```python
from build123d import *

# Parameters (mm, degrees)
SKETCH1_W           = 63.5
SKETCH1_H           = 63.5
BOSS_EXTRUDE1_DEPTH = 1.5875
FILLET1_R           = 0.508
FILLET2_R           = 3.175


with BuildPart() as part:
    # Sketch1 → Boss-Extrude1 (new body)
    with BuildSketch(Plane(origin=(0, 0, 0), x_dir=(1, 0, 0), z_dir=(0, 1, 0))):
        with Locations((31.75, 31.75)):
            Rectangle(SKETCH1_W, SKETCH1_H)
        with BuildLine():
            Line((24.384, 41.275), (24.384, 39.116))
            Line((24.384, 39.116), (21.388784565, 39.116))
            ThreePointArc((21.388784565, 39.116), (19.120478769, 30.298127151), (23.330551307, 22.225))
            Line((23.330551307, 22.225), (40.169448693, 22.225))
            ThreePointArc((40.169448693, 22.225), (40.739236377, 22.760763623), (41.275, 23.330551307))
            Line((41.275, 23.330551307), (41.275, 39.116))
            Line((41.275, 39.116), (39.116, 39.116))
            Line((39.116, 39.116), (39.116, 41.275))
            Line((39.116, 41.275), (24.384, 41.275))
        make_face(mode=Mode.SUBTRACT)
    extrude(amount=BOSS_EXTRUDE1_DEPTH)

    # Fillet1
    fillet1_edges = [part.edges().sort_by_distance(p)[0] for p in [
        (39.116, 0.79375, -39.116),
        (24.384, 0.79375, -39.116),
    ]]
    fillet(fillet1_edges, radius=FILLET1_R)

    # Fillet2
    fillet2_edges = [part.edges().sort_by_distance(p)[0] for p in [
        (0, 0.79375, -63.5),
        (63.5, 0.79375, -63.5),
        (63.5, 0.79375, 0),
        (0, 0.79375, 0),
    ]]
    fillet(fillet2_edges, radius=FILLET2_R)


solid = part.part
```
Model file for the job. Use its own axes, mm. A direction names the side the tool comes from. Give positions to 0.01 mm unless a question says otherwise; leave off trailing zeros. Loops run counter-clockwise (first coordinate to the right, second up) from the corner with the lowest first, then second, coordinate; pieces in that order, holes last. Notation, with made-up numbers: (80.25, 63) -> (118.25, 63) arc R33 cw to (118.25, 93) -> close; hole circle Ø1 at (80.25, 41.25). An arc over 180 degrees is marked (long way). Write each question's results on one line, items separated by ' | '.
(1) Tool access for faces 1 (the flat face through (31, 1, -63.5)), 2 (the flat face through (23, 1, -39.116)): list every direction of +Z, -Z, +X, -X, +Y, -Y with a clear straight run to the whole face (end or side of a thin tool).
Geometry results:
face 1: -Z, +X, -X, +Y, -Y | face 2: +Y, -Y
(2) Probe line 1 along Z through (x, y) = (34, 0.9) (3 decimals); line 2 along Z through (x, y) = (60.5, 0.55); line 3 along X through (y, z) = (0.9, -26.5) (3 decimals). List the from-to ranges inside material, lowest first.
Geometry results:
line 1: z = -63.5 to -41.275, -22.225 to 0 | line 2: z = -63.5 to 0 | line 3: x = 0 to 20.172, 41.275 to 63.5
(3) Cut at C-C on z = -36.5. List the corners of the cut face in (x, y) (1 decimal), and give its area (3 significant figures).
Geometry results:
outline: (0, 0) -> (20, 0) -> (20, 1.6) -> (0, 1.6) -> close; (41.3, 0) -> (63.5, 0) -> (63.5, 1.6) -> (41.3, 1.6) -> close | area: 67.0 mm²
(4) Flat gauge pin, fed straight in: pin 1 Ø1.5 at (x, z) = (26, -39) entering from -Y. Where does the tip first touch, or does it go through?
Geometry results:
pin 1: passes through
(5) Cut at A-A on y = 0.3. List the corners of the cut face in (x, z) (3 decimals), and give its area (3 significant figures).
Geometry results:
outline: (0, -60.325) arc R3.175 ccw to (3.175, -63.5) -> (60.325, -63.5) arc R3.175 ccw to (63.5, -60.325) -> (63.5, -3.175) arc R3.175 ccw to (60.325, 0) -> (3.175, 0) arc R3.175 ccw to (0, -3.175) -> close; hole (21.389, -39.116) -> (23.876, -39.116) arc R0.508 cw to (24.384, -39.624) -> (24.384, -41.275) -> (39.116, -41.275) -> (39.116, -39.624) arc R0.508 cw to (39.624, -39.116) -> (41.275, -39.116) -> (41.275, -23.331) arc R12.713 ccw to (40.169, -22.225) -> (23.331, -22.225) arc R12.713 ccw to start | area: 3,630 mm²
(6) Cut at B-B on x = 32. List the corners of the cut face in (y, z) (1 decimal).
Geometry results:
outline: (0, -63.5) -> (1.6, -63.5) -> (1.6, -41.3) -> (0, -41.3) -> close; (0, -22.2) -> (1.6, -22.2) -> (1.6, 0) -> (0, 0) -> close
(7) Pull direction Z, two halves, no side cores. Call faces 3 (the flat face through (41.275, 1, -31)), 4 (the cylindrical face through (62.55, 0.8, -62.59)), 5 (the flat face through (63.5, 1, -31)): released by +Z, released by -Z, zero draft, split by the parting line, or undercut.
Geometry results:
face 3: undercut | face 4: released by -Z | face 5: zero draft
